Could you check a few things on this model? Use its own coordinates, in mm. A direction names the side the tool comes from. Give positions to 0.01 mm unless a question says otherwise; leave off trailing zeros. Loops run counter-clockwise (first coordinate to the right, second up) from the corner with the lowest first, then second, coordinate; pieces in that order, holes last. Notation, with made-up numbers: M 64.25,-4 L 87.25,-4 A27 cw 87.25,22 Z; hole C 83.25,60.5 d5. An arc over 180 degrees is marked long. Answer in a Markdown table with one row per item. Add a question column.
1. If we section it at A-A on z = 3.5: List the corners of the cut face in (x, y) for me, then the cut area to 3 significant figures.
2. If we section it at B-B on y = -4.75: List the corners of the cut face in (x, z) for me, then the cut area to 3 significant figures.
3. If we section it at D-D on x = 0.75: List the corners of the cut face in (y, z) for me.
4. I'm going to push a flat-ended pin straight in: pin 1 Ø1.8 at (y, z) = (-5, 3.5) entering from -X. Where does the tip first touch, or does it pass through?
5. I need wall thicknesses on line 1 along X through (y, z) = (-1.15, 3.5); line 2 along Y through (x, z) = (3.5, 3.5); line 3 along X through (y, z) = (-3.5, 3.9). Which ranges of each line are inside material? Lowest first, please. Write a range as from..to.
6. Which directions (+Z, -Z, +X, -X, +Y, -Y) give clear straight access to the entire face, cutting with the end or side of a thin tool? Please do faces 1 (the cylindrical face through (3.58, -8.66, 3.54)), 2 (the flat face through (0, -1.412, 3)).
7. If we section it at C-C on z = 2.2: List the corners of the cut face in (x, y) for me.
8. Thinking about a two-plate mould opening in Z: for faces 3 (the cylindrical face through (-4.41, -1.17, 3.54)), 4 (the cylindrical face through (3.58, -4.7, 4.27)), 5 (the flat face through (3.338, -4, 4)), which applies, released by +Z, released by -Z, zero draft, split by the parting line, or undercut?
```python
from build123d import *

# Parameters (mm, degrees)
SKETCH_1_R      = 2.1
EXTRUDE_1_DEPTH = 1
SKETCH_2_R      = 2.1
EXTRUDE_2_DEPTH = 1
SCALE_2_SCALE   = 0.5
SCALE_1_SCALE   = 0.5
SCALE_3_SCALE   = 2


with BuildPart() as part:
    # Эскиз1 → Бобышка-Вытянуть1 (new body)
    with BuildSketch(Plane(origin=(0, 0, 0), x_dir=(1, 0, 0), z_dir=(0, 1, 0))):
        with BuildLine():
            Line((0, -7), (-7, -7))
            ThreePointArc((-7, -7), (-10.5, -3.5), (-7, 0))
            Line((-7, 0), (0, 0))
            Line((0, 0), (5, 0))
            Line((5, 0), (5, -7))
            Line((5, -7), (0, -7))
        make_face()
        with Locations(Location((-4, -3.5, 0), (0, 0, 270))):
            Circle(SKETCH_1_R, mode=Mode.SUBTRACT)
    extrude(amount=EXTRUDE_1_DEPTH)

    # Эскиз2 → Бобышка-Вытянуть2 (add)
    with BuildSketch(Plane(origin=(5, 0, 0), x_dir=(0, 0, -1), z_dir=(1, 0, 0))):
        with BuildLine():
            Line((0, -11), (0, 1))
            Line((0, 1), (-7, 1))
            Line((-7, 1), (-7, -11))
            ThreePointArc((-7, -11), (-3.5, -14.5), (0, -11))
        make_face()
        with Locations((-3.5, -8)):
            Circle(SKETCH_2_R, mode=Mode.SUBTRACT)
    extrude(amount=EXTRUDE_2_DEPTH)


with BuildPart() as part_1:
    # Масштаб2: scaled about (1.676803453, -2.823196547, 3.5)
    add(part.part.scale(SCALE_2_SCALE).moved(Location((0.838401726, -1.411598273, 1.75))))


with BuildPart() as part_2:
    # Масштаб1: scaled about (1.676803453, -2.823196547, 3.5)
    add(part_1.part.scale(SCALE_1_SCALE).moved(Location((0.838401726, -1.411598273, 1.75))))


with BuildPart() as part_3:
    # Масштаб3: scaled about (1.676803453, -2.823196547, 3.5)
    add(part_2.part.scale(SCALE_3_SCALE).moved(Location((-1.676803453, 2.823196547, -3.5))))


solid = part_3.part
```
Results:
| question | item | result |
|---|---|---|
| 1 | outline | M -4.41,-1.41 L -2.21,-1.41 L -2.21,-0.91 L -4.41,-0.91 Z; M -0.11,-1.41 L 3.34,-1.41 L 3.34,-4.36 L 3.84,-4.36 L 3.84,-0.91 L -0.11,-0.91 Z; M 3.34,-8.66 L 3.84,-8.66 L 3.84,-6.46 L 3.34,-6.46 Z |
| 1 | area | 5.65 mm2 |
| 2 | outline | M 3.34,1.75 L 3.84,1.75 L 3.84,2.68 L 3.34,2.68 Z; M 3.34,4.32 L 3.84,4.32 L 3.84,5.25 L 3.34,5.25 Z |
| 2 | area | 0.935 mm2 |
| 3 | outline | M -1.41,1.75 L -0.91,1.75 L -0.91,5.25 L -1.41,5.25 Z |
| 4 | pin 1 | x = 3.34 |
| 5 | line 1 | -4.41..-2.21, -0.11..3.84 |
| 5 | line 2 | -8.66..-6.46, -4.36..-0.91 |
| 5 | line 3 | 3.34..3.84 |
| 6 | face 1 | +X, -X, -Y |
| 6 | face 2 | +Z, -Z, -X, -Y |
| 7 | outline | M -3.83,-1.41 L 3.34,-1.41 L 3.34,-8.08 L 3.84,-8.08 L 3.84,-0.91 L -3.83,-0.91 Z |
| 8 | face 3 | split by the parting line |
| 8 | face 4 | undercut |
| 8 | face 5 | zero draft |
